```python
from build123d import *

# Parameters (mm, degrees)
F0_W     = 19.05
F0_H     = 82.530156
F0_R     = 3.175
F1_DEPTH = 12.7
F2_W     = 15.875
F2_H     = 9.525
F3_DEPTH = 19.051


with BuildPart() as f1:
    # F0 (on Top) → F1 (new body)
    with BuildSketch(Plane.XY):
        Rectangle(F0_W, F0_H)
        with Locations((0, -25.4)):
            Circle(F0_R, mode=Mode.SUBTRACT)
        with Locations((0, 25.4)):
            Circle(F0_R, mode=Mode.SUBTRACT)
    extrude(amount=F1_DEPTH)

    # F2 (on face) → F3 (cut, through all)
    with BuildSketch(Plane(origin=(-9.525, 0, 0), x_dir=(0, -1, 0), z_dir=(-1, 0, 0))):
        Rectangle(F2_W, F2_H)
    extrude(amount=-F3_DEPTH, mode=Mode.SUBTRACT)


solid = f1.part
```
The listing builds one solid part. Answer for the finished solid, in the listing's coordinates (mm). A direction names the side the tool comes from. Give positions to 0.01 mm unless a question says otherwise; leave off trailing zeros. Write each loop counter-clockwise with the first axis right and the second up, starting at its lowest first coordinate (ties: lowest second). Pieces come first, ordered by that corner, then holes. Notation, with made-up numbers: (89, 57.5) -> (134, 57.5) arc R27 cw to (134, 75.5) -> close; hole circle Ø4 at (-38.75, -9.75). An arc over 180 degrees is marked (long way). Use one line per item in the form item = value.
1) Straight lines are drawn through the part: probe 1 along Y at (x, z) = (0, 8.25) (3 decimals); probe 2 along Y at (x, z) = (-5.25, 3); probe 3 along Y at (x, z) = (1.25, 5). For each, find the intervals that lie inside material, in ascending order.
Result:
probe_1 = -41.265 to -28.575, -22.225 to 22.225, 28.575 to 41.265
probe_2 = -41.27 to -7.94, 7.94 to 41.27
probe_3 = -41.27 to -28.32, -22.48 to 22.48, 28.32 to 41.27
2) Section A-A on y = -25.4 is taken. Write down the section's boundary in (x, z) (3 decimals), plus the area to 3 significant figures.
Result:
outline = (-9.525, 0) -> (-3.175, 0) -> (-3.175, 12.7) -> (-9.525, 12.7) -> close; (3.175, 0) -> (9.525, 0) -> (9.525, 12.7) -> (3.175, 12.7) -> close
area = 161 mm²
3) Section C-C on x = -6 is taken. Write down the section's boundary in (y, z).
Result:
outline = (-41.27, 0) -> (-7.94, 0) -> (-7.94, 4.76) -> (7.94, 4.76) -> (7.94, 0) -> (41.27, 0) -> (41.27, 12.7) -> (-41.27, 12.7) -> close
4) Section B-B on z = 1.75 is taken. Count the separate pieces of the cut face and the enclosed holes in it, plus the area to 3 significant figures.
Result:
separate_pieces = 2
enclosed_holes = 2
area = 1,210 mm²
5) Section D-D on z = 12 is taken. Write down the section's boundary in (x, y) (3 decimals), plus the area to 3 significant figures.
Result:
outline = (-9.525, -41.265) -> (9.525, -41.265) -> (9.525, 41.265) -> (-9.525, 41.265) -> close; hole circle Ø6.35 at (0, -25.4); hole circle Ø6.35 at (0, 25.4)
area = 1,510 mm²
6) Each of these flat-tipped pins is pushed along its axis until it touches: P1, Ø5.5, axis at x = 0, y = -25.4, coming from the -Z side (3 decimals); P2, Ø8, axis at x = 3.5, y = 0.5, coming from the -Z side. Where does it stop, or does it pass through?
Result:
P1 = through
P2 = 4.76
7) For a pull along Y with two mould halves and no side action, classify faces 1 (the flat face through (0, -41.265, 6)), 2 (the flat face through (0, -21, 0)), 3 (the cylindrical face through (-0.41, -22.25, 6.26)) as +Y half, -Y half, draft (parallel to the pull), parting line (faces both ways), or undercut.
Result:
face_1 = -Y half
face_2 = draft
face_3 = undercut
8) A tool of negligible diameter and unlimited length cuts with its end or side. For faces 4 (the flat face through (0, 0, 4.762)), 5 (the flat face through (-9.525, -1, 6)), from which of +Z, -Z, +X, -X, +Y, -Y can it reach the whole face along a straight path? Write none if from no direction.
Result:
face_4 = -Z, +X, -X
face_5 = +Z, -Z, -X, +Y, -Y
